The listing builds one solid part. Answer for the finished solid, in the listing's coordinates (mm). Give positions to 0.01 mm unless a question says otherwise; leave off trailing zeros. Write each loop counter-clockwise with the first axis right and the second up, starting at its lowest first coordinate (ties: lowest second). Pieces come first, ordered by that corner, then holes.
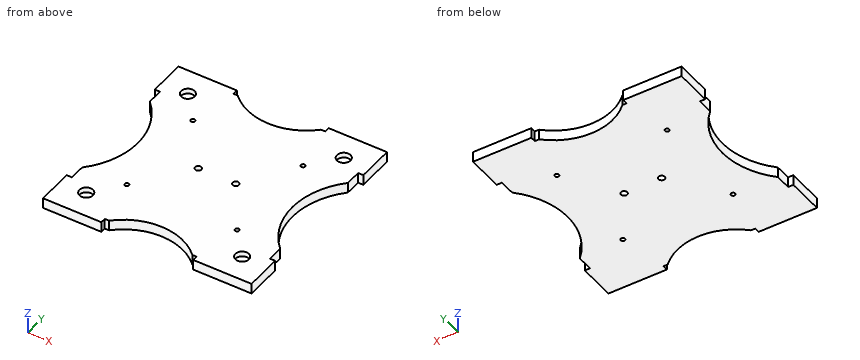
```python
from build123d import *

# Parameters (mm, degrees)
SKETCH1_R           = 1.5
BOSS_EXTRUDE1_DEPTH = 10
SKETCH2_R           = 2
CUT_EXTRUDE1_DEPTH  = 10
BOSS_EXTRUDE2_START = -10
SKETCH3_R           = 1.5
BOSS_EXTRUDE2_DEPTH = 10
BOSS_EXTRUDE3_START = -10
SKETCH5_R           = 1.5
BOSS_EXTRUDE3_DEPTH = 10
SKETCH6_R           = 6.5
CUT_EXTRUDE3_DEPTH  = 5
SKETCH8_R           = 3
CUT_EXTRUDE4_DEPTH  = 10


with BuildPart() as part:
    # Sketch1 → Boss-Extrude1 (new body)
    with BuildSketch(Plane.XY):
        with BuildLine():
            ThreePointArc((-40, 95), (0, 78.431457505), (40, 95))
            Line((40, 95), (44.1, 95))
            Line((44.1, 95), (44.1, 100))
            Line((44.1, 100), (100, 100))
            Line((100, 100), (100, 65))
            Line((100, 65), (95, 65))
            Line((95, 65), (95, 50))
            ThreePointArc((95, 50), (74.289321881, 0), (95, -50))
            Line((95, -50), (95, -65))
            Line((95, -65), (100, -65))
            Line((100, -65), (100, -100))
            Line((100, -100), (44.1, -100))
            Line((44.1, -100), (44.1, -95))
            Line((44.1, -95), (40, -95))
            ThreePointArc((40, -95), (0, -78.431457505), (-40, -95))
            Line((-40, -95), (-44.1, -95))
            Line((-44.1, -95), (-44.1, -100))
            Line((-44.1, -100), (-100, -100))
            Line((-100, -100), (-100, -65))
            Line((-100, -65), (-95, -65))
            Line((-95, -65), (-95, -50))
            ThreePointArc((-95, -50), (-74.289321881, 0), (-95, 50))
            Line((-95, 50), (-95, 65))
            Line((-95, 65), (-100, 65))
            Line((-100, 65), (-100, 100))
            Line((-100, 100), (-44.1, 100))
            Line((-44.1, 100), (-44.1, 95))
            Line((-44.1, 95), (-40, 95))
        make_face()
        with Locations((74.775, -75)):
            Circle(SKETCH1_R, mode=Mode.SUBTRACT)
        with Locations((-74.775, -75)):
            Circle(SKETCH1_R, mode=Mode.SUBTRACT)
        with Locations((-74.775, 75)):
            Circle(SKETCH1_R, mode=Mode.SUBTRACT)
        with Locations((74.775, 75)):
            Circle(SKETCH1_R, mode=Mode.SUBTRACT)
    extrude(amount=BOSS_EXTRUDE1_DEPTH)

    # Sketch2 → Cut-Extrude1 (cut)
    with BuildSketch(Plane.XY.offset(10)):
        with Locations((52.87, -48.68)):
            Circle(SKETCH2_R)
        with Locations((-52.87, -48.68)):
            Circle(SKETCH2_R)
        with Locations((52.87, 48.68)):
            Circle(SKETCH2_R)
        with Locations((-52.87, 48.68)):
            Circle(SKETCH2_R)
    extrude(amount=-CUT_EXTRUDE1_DEPTH, mode=Mode.SUBTRACT)

    # Sketch3 → Boss-Extrude2 (add)
    with BuildSketch(Plane.XY.offset(10).offset(BOSS_EXTRUDE2_START)):
        with Locations((74.775, -75)):
            Circle(SKETCH3_R)
    extrude(amount=BOSS_EXTRUDE2_DEPTH)

    # Sketch5 → Boss-Extrude3 (add)
    with BuildSketch(Plane.XY.offset(10).offset(BOSS_EXTRUDE3_START)):
        with Locations((-74.775, -75)):
            Circle(SKETCH5_R)
        with Locations((-74.775, 75)):
            Circle(SKETCH5_R)
        with Locations((74.775, 75)):
            Circle(SKETCH5_R)
    extrude(amount=BOSS_EXTRUDE3_DEPTH)

    # Sketch6 → Cut-Extrude3 (cut)
    with BuildSketch(Plane.XY.offset(10)):
        with Locations((-74.775, 75)):
            Circle(SKETCH6_R)
        with Locations((74.775, 75)):
            Circle(SKETCH6_R)
        with Locations((74.775, -75)):
            Circle(SKETCH6_R)
        with Locations((-74.775, -75)):
            Circle(SKETCH6_R)
    extrude(amount=-CUT_EXTRUDE3_DEPTH, mode=Mode.SUBTRACT)

    # Sketch8 → Cut-Extrude4 (cut)
    with BuildSketch(Plane.XY.offset(10)):
        with Locations((20, 0)):
            Circle(SKETCH8_R)
        with Locations((-16, 0)):
            Circle(SKETCH8_R)
    extrude(amount=-CUT_EXTRUDE4_DEPTH, mode=Mode.SUBTRACT)


solid = part.part
```
Item 1: A cutting plane is placed at D-D, the plane y = -21. Give the vertices of the cut face in (x, z), plus the area to 3 significant figures.
Conclusion:
outline: (-77.48, 0) - (77.48, 0) - (77.48, 10) - (-77.48, 10) - close
area: 1,550 mm2
Item 2: A cutting plane is placed at B-B, the plane y = 0. Give the vertices of the cut face in (x, z).
Conclusion:
outline: (-74.29, 0) - (-19, 0) - (-19, 10) - (-74.29, 10) - close; (-13, 0) - (17, 0) - (17, 10) - (-13, 10) - close; (23, 0) - (74.29, 0) - (74.29, 10) - (23, 10) - close
Item 3: A cutting plane is placed at A-A, the plane z = 3.5. Count the separate pieces of the cut face and the enclosed holes in it, plus the area to 3 significant figures.
Conclusion:
separate pieces: 1
enclosed holes: 6
area: 33,000 mm2
Item 4: A cutting plane is placed at C-C, the plane x = -71. Give the vertices of the cut face in (y, z), plus the area to 3 significant figures.
Conclusion:
outline: (-100, 0) - (100, 0) - (100, 10) - (80.29, 10) - (80.29, 5) - (69.71, 5) - (69.71, 10) - (-69.71, 10) - (-69.71, 5) - (-80.29, 5) - (-80.29, 10) - (-100, 10) - close
area: 1,890 mm2
Item 5: Each of these flat-tipped pins is pushed along its axis until it touches: P1, Ø1, axis at y = 33.5, z = 1.5, coming from the -X side; P2, Ø3.5, axis at x = 52.87, y = 48.68, coming from the +Z side; P3, Ø6.5, axis at x = 75.5, y = -72, coming from the +Z side; P4, Ø4.5, axis at x = 41.5, z = 6.5, coming from the +Y side. Where does it stop, or does it pass through?
Conclusion:
P1: stops at x = -83
P2: passes through
P3: stops at z = 5
P4: stops at y = 95
Item 6: Consider probe 1 along Y at (x, z) = (-52.87, 7.25); probe 2 along X at (y, z) = (2, 8.25); probe 3 along X at (y, z) = (-69.5, 5.5). Determine where each line is inside the solid, lowest interval first.
Conclusion:
probe 1: y = -100 to -50.68, -46.68 to 46.68, 50.68 to 100
probe 2: x = -74.32 to -18.24, -13.76 to 17.76, 22.24 to 74.32
probe 3: x = -100 to -78.24, -71.31 to 71.31, 78.24 to 100
